Autodesk Inventor part; units mm, degrees
ref_plane "YZ Plane" through (0, 0, 0) normal (1, 0, 0) x (0, 1, 0)
ref_plane "XZ Plane" through (0, 0, 0) normal (0, 1, 0) x (-1, 0, 0)
ref_plane "XY Plane" through (0, 0, 0) normal (0, 0, 1) x (1, 0, 0)
sketch "Sketch1" plane through (0, 0, 0) normal (0, 1, 0) x (-1, 0, 0)
  line L0 (57.15, 25.4) -> (44.45, 25.4)
  line L1 (44.45, 25.4) -> (44.45, 0)
  line L2 (44.45, 0) -> (57.15, 0)
  line L3 (57.15, 0) -> (57.15, 25.4)
  line L4 (-44.45, 25.4) -> (-57.15, 25.4)
  line L5 (-57.15, 25.4) -> (-57.15, 0)
  line L6 (-57.15, 0) -> (-44.45, 0)
  line L7 (-44.45, 0) -> (-44.45, 25.4)
  line L8 (44.45, 25.4) -> (-44.45, 25.4) construction
  point P0 (0, 0)
  dimension "d0" = 12.7
  dimension "d1" = 25.4
  dimension "d2" = 114.3
  dimension "d3" = 57.15
extrude "Extrusion1" add sketch "Sketch1" along normal blind 2.54
sketch "Sketch2" plane through (57.15, 0, 0) normal (0, 0, -1) x (-1, 0, 0)
  line L0 (0, 0.9525) -> (12.7, 0.9525)
  line L1 (12.7, 0.9525) -> (12.7, 73.3425)
  line L2 (12.7, 73.3425) -> (0, 73.3425)
  line L3 (0, 73.3425) -> (0, 0.9525)
  line L4 (101.6, 0) -> (114.3, 0)
  line L5 (114.3, 0) -> (114.3, 72.39)
  line L6 (114.3, 72.39) -> (101.6, 72.39)
  line L7 (101.6, 72.39) -> (101.6, 0)
  line L8 (12.7, 0) -> (12.7, 2.54)
  point P0 (57.15, 0)
  dimension "d6" = 12.7
  dimension "d7" = 12.7
  dimension "d8" = 12.7
  dimension "d9" = 72.39
extrude "Extrusion2" add sketch "Sketch2" against normal blind 2.54
sketch "Sketch3" plane through (57.15, 0, 2.54) normal (0, 0, 1) x (1, 0, 0)
  line L0 (-114.3, 72.39) -> (-114.3, 2.54)
  line L1 (0, 2.54) -> (0, 73.3425)
  line L2 (-114.3, 72.39) -> (0, 72.39)
  line L3 (0, 72.39) -> (0, 46.99)
  line L4 (0, 46.99) -> (-114.3, 46.99)
  line L5 (-114.3, 46.99) -> (-114.3, 72.39)
  point P0 (-57.15, 0)
  point P1 (0, 72.39)
  point P2 (0, 3.81)
  dimension "d12" = 25.4
extrude "Extrusion3" add sketch "Sketch3" along normal blind 2.54
sketch "Sketch4" plane through (57.15, 0, 5.08) normal (0, 0, 1) x (1, 0, 0)
  circle A0 centre (-107.95, 59.69) radius 2.54
  circle A1 centre (-6.35, 59.69) radius 2.54
  line L0 (-114.3, 72.39) -> (-114.3, 46.99)
  line L1 (-114.3, 59.69) -> (-107.95, 59.69)
  line L2 (-107.95, 59.69) -> (-6.35, 59.69)
  line L3 (-6.35, 59.69) -> (0, 59.69)
  line L4 (0, 46.99) -> (0, 72.39)
  point P0 (-57.15, 0)
  dimension "d15" = 5.08
  dimension "d16" = 6.35
extrude "Extrusion4" add sketch "Sketch4" along normal blind 2.54
sketch "Sketch5" plane through (0, 2.54, 0) normal (0, 1, 0) x (1, 0, 0)
  circle A0 centre (-50.8, -20.32) radius 2.54
  circle A1 centre (50.8, -20.32) radius 2.54
  line L0 (-57.15, -25.4) -> (-44.45, -25.4)
  line L1 (-50.8, -25.4) -> (-50.8, 0) construction
  line L2 (44.45, -25.4) -> (57.15, -25.4)
  line L3 (50.8, -25.4) -> (50.8, 0) construction
  point P0 (0, 0)
  dimension "d19" = 5.08
  dimension "d20" = 5.08
  dimension "d21" = 5.08
extrude "Extrusion5" add sketch "Sketch5" along normal blind 2.54
equation "\"d21\" = d20"
properties part number "Frame"
Geometry: final body of the model. Coordinates: model frame, mm. A direction names the side the tool comes from. Round coordinates to 2 decimals unless told otherwise and drop trailing zeros. Loops run counter-clockwise (first coordinate to the right, second up) from the corner with the lowest first, then second, coordinate; pieces in that order, holes last.
Q1. Pin query (flat end, axial travel): P1, Ø4, axis at x = -50, y = 14.5, coming from the +Z side; P2, Ø1.5, axis at x = 50, y = 59.5, coming from the +Z side; P3, Ø14, axis at x = -54, z = 15.5, coming from the +Y side. Return the tip coordinate at first contact, or that it passes through.
Q2. Material intervals for L1, parallel to Z at x = 39, y = 68; L2, parallel to Z at x = 45.5, y = 48.5; L3, parallel to Y at x = -49, z = 23.5, sorted ascending.
Q3. Section A-A on z = 15.25. Return loops of the section in (x, y), plus the area to 3 significant figures.
Q4. Section C-C on x = -46. Return loops of the section in (y, z), plus the area to 3 significant figures.
Q5. Section D-D on y = 63.5. Return loops of the section in (x, z), plus the area to 3 significant figures.
Q6. Access query for faces 4 (the flat face through (-1, 60, 2.54)), 5 (the flat face through (-51, 5.08, 20)), 6 (the flat face through (1, 46.99, 4)), 7 (the cylindrical face through (53.146, 3.792, 19.347)). Directions: +Z, -Z, +X, -X, +Y, -Y. A direction counts if a zero-diameter tool reaches every point of the face in a straight line with its end or side. Return the directions, or none.
Q7. Pull-direction query (Y, two-part tool) for faces 1 (the flat face through (51, 60, 7.62)), 2 (the flat face through (51, 2.54, 14)), 3 (the flat face through (51, 5.08, 20)); classes: released by +Y, released by -Y, zero draft, split by the parting line, or undercut.
Evaluation:
1. P1: stops at z = 2.54
1. P2: stops at z = 7.62
1. P3: stops at y = 5.08
2. L1: z = 2.54 to 5.08
2. L2: z = 0 to 5.08
2. L3: y = 0 to 2.54
3. outline: (-57.15, 0) - (-44.45, 0) - (-44.45, 2.54) - (-57.15, 2.54) - close; (44.45, 0) - (57.15, 0) - (57.15, 2.54) - (44.45, 2.54) - close
3. area: 64.5 mm2
4. outline: (0, 0) - (72.39, 0) - (72.39, 5.08) - (46.99, 5.08) - (46.99, 2.54) - (2.54, 2.54) - (2.54, 25.4) - (0, 25.4) - close
4. area: 306 mm2
5. outline: (-57.15, 0) - (-44.45, 0) - (-44.45, 2.54) - (44.45, 2.54) - (44.45, 0) - (57.15, 0) - (57.15, 5.08) - (-57.15, 5.08) - close
5. area: 355 mm2
6. face 4: -Z, +Y, -Y
6. face 5: +Z, +X, -X, +Y
6. face 6: +Z, +X, -X
6. face 7: +Y
7. face 1: zero draft
7. face 2: undercut
7. face 3: released by +Y
